Design review of the part built by this model. Coordinates are the model's own, in mm. A direction names the side the tool comes from. Coordinates: 2 decimals unless noted, no trailing zeros. Write each loop counter-clockwise with the first axis right and the second up, starting at its lowest first coordinate (ties: lowest second). Pieces come first, ordered by that corner, then holes.
Q1. Take a section at B-B (z = -167). Give the boundary of the cut face in (x, y), and give its area (3 significant figures).
Q2. For probe 1 along X at (y, z) = (2.35, -178); probe 2 along Z at (x, y) = (118.5, 0.75); probe 3 along Z at (x, y) = (104.7, 0.7), list the stretches that pass through material, from the lowest coordinate up.
Q3. Insertion check: pin 1 (2.5 mm diameter, centred on x = 104.7, z = -177.8, fed in from -Y); pin 2 (5 mm diameter, centred on x = 6.5, z = -193.5, fed in from -Y); pin 3 (0.8 mm diameter, centred on y = 0.5, z = -92.5, fed in from -X). Each pin has a flat end and moves straight along its axis. Give the tip position at first contact, or say it passes through.
Q4. Take a section at C-C (z = -136.5). Give the boundary of the cut face in (x, y), and give its area (4 significant figures).
Q5. Take a section at A-A (y = 0.75). State how many separate pieces and enclosed holes the cut face has, and give its area (3 significant figures).
Q6. Machinability: for faces 1 (the flat face through (62, 2.5, -101)), 2 (the flat face through (12.3, 1.2, -159)), 3 (the flat face through (112.3, 1.2, -158.6)), which of the approach directions +Z, -Z, +X, -X, +Y, -Y give a long, thin tool a straight path to every point of the face, cutting with its end or side? Answer none if there is none.
```python
from build123d import *

# Parameters (mm, degrees)
SKETCH1_R           = 1.5
SKETCH1_W           = 8.4
SKETCH1_H           = 16
BOSS_EXTRUDE1_DEPTH = 2.5


with BuildPart() as part:
    # Sketch1 → Boss-Extrude1 (new body)
    with BuildSketch(Plane(origin=(0, 0, 0), x_dir=(1, 0, 0), z_dir=(0, 1, 0))):
        Polygon((0, 0), (125, 0), (125, 28.7), (100, 53.7), (100, 146.3), (125, 171.3), (125, 200), (0, 200), (0, 171.3), (25, 146.3), (25, 53.7), (0, 28.7), align=None)
        with Locations(Location((6.5, 6.5, 0), (0, 0, 270))):
            Circle(SKETCH1_R, mode=Mode.SUBTRACT)
        with Locations(Location((6.5, 22.2, 0), (0, 0, 270))):
            Circle(SKETCH1_R, mode=Mode.SUBTRACT)
        with Locations(Location((20.3, 6.5, 0), (0, 0, 270))):
            Circle(SKETCH1_R, mode=Mode.SUBTRACT)
        with Locations(Location((20.3, 22.2, 0), (0, 0, 270))):
            Circle(SKETCH1_R, mode=Mode.SUBTRACT)
        with Locations(Location((104.7, 6.5, 0), (0, 0, 90))):
            Circle(SKETCH1_R, mode=Mode.SUBTRACT)
        with Locations(Location((118.5, 6.5, 0), (0, 0, 90))):
            Circle(SKETCH1_R, mode=Mode.SUBTRACT)
        with Locations(Location((104.7, 22.2, 0), (0, 0, 90))):
            Circle(SKETCH1_R, mode=Mode.SUBTRACT)
        with Locations(Location((118.5, 22.2, 0), (0, 0, 90))):
            Circle(SKETCH1_R, mode=Mode.SUBTRACT)
        with Locations(Location((118.5, 177.8, 0), (0, 0, 270))):
            Circle(SKETCH1_R, mode=Mode.SUBTRACT)
        with Locations(Location((118.5, 193.5, 0), (0, 0, 270))):
            Circle(SKETCH1_R, mode=Mode.SUBTRACT)
        with Locations(Location((104.7, 193.5, 0), (0, 0, 270))):
            Circle(SKETCH1_R, mode=Mode.SUBTRACT)
        with Locations(Location((104.7, 177.8, 0), (0, 0, 270))):
            Circle(SKETCH1_R, mode=Mode.SUBTRACT)
        with Locations(Location((20.3, 193.5, 0), (0, 0, 90))):
            Circle(SKETCH1_R, mode=Mode.SUBTRACT)
        with Locations(Location((20.3, 177.8, 0), (0, 0, 90))):
            Circle(SKETCH1_R, mode=Mode.SUBTRACT)
        with Locations(Location((6.5, 193.5, 0), (0, 0, 90))):
            Circle(SKETCH1_R, mode=Mode.SUBTRACT)
        with Locations(Location((6.5, 177.8, 0), (0, 0, 90))):
            Circle(SKETCH1_R, mode=Mode.SUBTRACT)
        with Locations((56, 14.35)):
            Rectangle(SKETCH1_W, SKETCH1_H, mode=Mode.SUBTRACT)
        with Locations((69, 14.35)):
            Rectangle(SKETCH1_W, SKETCH1_H, mode=Mode.SUBTRACT)
    extrude(amount=BOSS_EXTRUDE1_DEPTH)


solid = part.part
```
Response:
1. outline: (4.3, 0) - (120.7, 0) - (120.7, 2.5) - (4.3, 2.5) - close
1. area: 291 mm2
2. probe 1: x = 0 to 5.01, 7.99 to 18.81, 21.79 to 103.21, 106.19 to 117.01, 119.99 to 125
2. probe 2: z = -200 to -195, -192 to -179.3, -176.3 to -164.8, -35.2 to -23.7, -20.7 to -8, -5 to 0
2. probe 3: z = -200 to -195, -192 to -179.3, -176.3 to -151, -49 to -23.7, -20.7 to -8, -5 to 0
3. pin 1: passes through
3. pin 2: stops at y = 0
3. pin 3: stops at x = 25
4. outline: (25, 0) - (100, 0) - (100, 2.5) - (25, 2.5) - close
4. area: 187.5 mm2
5. separate pieces: 1
5. enclosed holes: 18
5. area: 18,700 mm2
6. face 1: +Z, -Z, +X, -X, +Y
6. face 2: -X, +Y, -Y
6. face 3: +X, +Y, -Y
